```python
from build123d import *

# Parameters (mm, degrees)
F0_R     = 4.7625
F1_DEPTH = 18.8087
F2_R     = 4.7625
F3_DEPTH = 12.7
F4_DEPTH = 6.35


with BuildPart() as f1:
    # F0 (on Top) → F1 (new body)
    with BuildSketch(Plane.XY):
        Circle(F0_R)
    extrude(amount=F1_DEPTH)

    # F2 (on face) → F3 (join)
    with BuildSketch(Plane.XY.offset(18.8087)):
        with BuildLine():
            ThreePointArc((7.493, 2.3622), (6.563064, 4.607264), (4.318, 5.5372))
            Line((4.318, 5.5372), (-4.318, 5.5372))
            ThreePointArc((-4.318, 5.5372), (-6.563064, 4.607264), (-7.493, 2.3622))
            Line((-7.493, 2.3622), (-7.493, -2.3622))
            ThreePointArc((-7.493, -2.3622), (-6.563064, -4.607264), (-4.318, -5.5372))
            Line((-4.318, -5.5372), (4.318, -5.5372))
            ThreePointArc((4.318, -5.5372), (6.563064, -4.607264), (7.493, -2.3622))
            Line((7.493, -2.3622), (7.493, 2.3622))
        make_face()
        Circle(F2_R, mode=Mode.SUBTRACT)
        Circle(F2_R)
    extrude(amount=F3_DEPTH)

    # F2 (on face) → F4 (join)
    with BuildSketch(Plane.XY.offset(18.8087)):
        with BuildLine():
            Line((8.001, -2.3622), (8.001, 2.3622))
            ThreePointArc((8.001, 2.3622), (6.922274, 4.966474), (4.318, 6.0452))
            Line((4.318, 6.0452), (-4.318, 6.0452))
            ThreePointArc((-4.318, 6.0452), (-6.922274, 4.966474), (-8.001, 2.3622))
            Line((-8.001, 2.3622), (-8.001, -2.3622))
            ThreePointArc((-8.001, -2.3622), (-6.922274, -4.966474), (-4.318, -6.0452))
            Line((-4.318, -6.0452), (4.318, -6.0452))
            ThreePointArc((4.318, -6.0452), (6.922274, -4.966474), (8.001, -2.3622))
        make_face()
        with BuildLine():
            Line((-4.318, 5.5372), (4.318, 5.5372))
            ThreePointArc((4.318, 5.5372), (6.563064, 4.607264), (7.493, 2.3622))
            Line((7.493, 2.3622), (7.493, -2.3622))
            ThreePointArc((7.493, -2.3622), (6.563064, -4.607264), (4.318, -5.5372))
            Line((4.318, -5.5372), (-4.318, -5.5372))
            ThreePointArc((-4.318, -5.5372), (-6.563064, -4.607264), (-7.493, -2.3622))
            Line((-7.493, -2.3622), (-7.493, 2.3622))
            ThreePointArc((-7.493, 2.3622), (-6.563064, 4.607264), (-4.318, 5.5372))
        make_face(mode=Mode.SUBTRACT)
    extrude(amount=F4_DEPTH)


solid = f1.part
```
Input: part model. Units: mm. Frame: model coordinates. A direction names the side the tool comes from. Coordinates: 2 decimals unless noted, no trailing zeros. Write each loop counter-clockwise with the first axis right and the second up, starting at its lowest first coordinate (ties: lowest second). Pieces come first, ordered by that corner, then holes. Notation, with made-up numbers: (15, 0) -> (55, 0) arc R14 ccw to (55, 8) -> close; hole circle Ø7 at (69, -23.75). An arc over 180 degrees is marked (long way). Write each question's results on one line, items separated by ' | '.
Item 1: Pin query (flat end, axial travel): pin 1 Ø1.9 at (x, z) = (-1.5, 28) entering from -Y; pin 2 Ø2.5 at (y, z) = (0, 28) entering from +X; pin 3 Ø2 at (y, z) = (4, 19.5) entering from +X. Return the tip coordinate at first contact, or that it passes through.
Conclusion:
pin 1: stops at y = -5.54 | pin 2: stops at x = 7.49 | pin 3: stops at x = 7.95
Item 2: Section query D-D on x = 5.75. Return loops of the section in (y, z), plus the area to 3 significant figures.
Conclusion:
outline: (-5.76, 18.81) -> (5.76, 18.81) -> (5.76, 25.16) -> (5.2, 25.16) -> (5.2, 31.51) -> (-5.2, 31.51) -> (-5.2, 25.16) -> (-5.76, 25.16) -> close | area: 139 mm^2
Item 3: Material intervals for probe 1 along Y at (x, z) = (4.5, 26); probe 2 along Z at (x, y) = (6.5, -0.75); probe 3 along X at (y, z) = (-0.25, 11), sorted ascending.
Conclusion:
probe 1: y = -5.53 to 5.53 | probe 2: z = 18.81 to 31.51 | probe 3: x = -4.76 to 4.76
Item 4: Set-up query: faces 1 (the flat face through (0, 5.8, 25.159)), 2 (the flat face through (0, -5.537, 28)), 3 (the flat face through (-5, 0, 18.809)), 4 (the flat face through (0, 5.537, 28)). Return all of +Z, -Z, +X, -X, +Y, -Y with unobstructed straight access to the full face (end or side cutting, diameter ignored); none if empty.
Conclusion:
face 1: +Z | face 2: +Z, +X, -X, -Y | face 3: -Z | face 4: +Z, +X, -X, +Y
Item 5: Section query C-C on z = 14.5. Return loops of the section in (x, y) (1 decimal).
Conclusion:
outline: circle Ø9.5 at (0, 0)
Item 6: Section query A-A on y = 0. Return loops of the section in (x, z), plus the area to 3 significant figures.
Conclusion:
outline: (-8, 18.81) -> (-4.76, 18.81) -> (-4.76, 0) -> (4.76, 0) -> (4.76, 18.81) -> (8, 18.81) -> (8, 25.16) -> (7.49, 25.16) -> (7.49, 31.51) -> (-7.49, 31.51) -> (-7.49, 25.16) -> (-8, 25.16) -> close | area: 376 mm^2
Item 7: Section query B-B on x = 0. Return loops of the section in (y, z).
Conclusion:
outline: (-6.05, 18.81) -> (-4.76, 18.81) -> (-4.76, 0) -> (4.76, 0) -> (4.76, 18.81) -> (6.05, 18.81) -> (6.05, 25.16) -> (5.54, 25.16) -> (5.54, 31.51) -> (-5.54, 31.51) -> (-5.54, 25.16) -> (-6.05, 25.16) -> close
